Can you work these out from the model? Positions are in its coordinate system, mm. Face numbers are marked on the shaded views. A direction names the side the tool comes from. Give positions to 0.01 mm unless a question says otherwise; leave off trailing zeros. Order: outer loops, then holes, each group sorted by start corner. A loop starts at its lowest first (then second) coordinate and runs counter-clockwise, first axis right, second up. Notation, with made-up numbers: M 39,68 L 61,68 A16 ccw 61,91 Z; hole C 25.25,83 d6. An arc over 180 degrees is marked long. Answer as a JSON object with one key per item and string values.
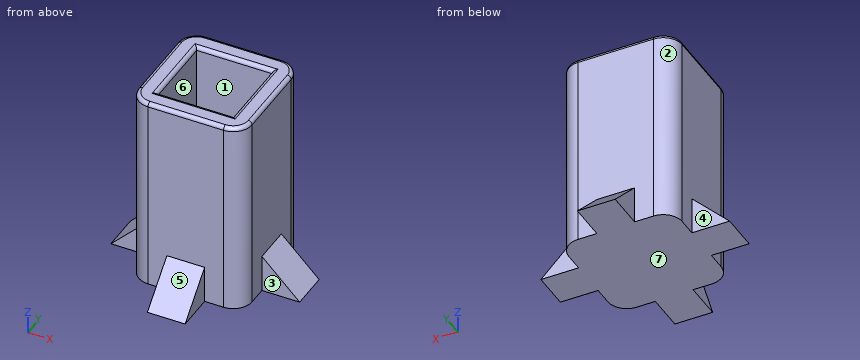
```python
from build123d import *

# Parameters (mm, degrees)
F0_W            = 30
F0_H            = 30
F1_DEPTH        = 3
F2_W            = 30
F2_H            = 30
F2_W_2          = 20
F2_H_2          = 20
F3_DEPTH        = 50
F4_R            = 5
F5_R            = 1
F7_DEPTH        = 5
F7_DEPTH_BACK   = 5
F7_COPIES_COUNT = 4


# Not quite as in the source:
# - a pattern or mirror of a feature is missing from the dataset's text; its kind, count and spacing are read off the source's solid


with BuildPart() as f1:
    # F0 (on Top) → F1 (new body)
    with BuildSketch(Plane.XY):
        Rectangle(F0_W, F0_H)
    extrude(amount=F1_DEPTH)

    # F2 (on face) → F3 (join)
    with BuildSketch(Plane.XY.offset(3)):
        Rectangle(F2_W, F2_H)
        Rectangle(F2_W_2, F2_H_2, mode=Mode.SUBTRACT)
    extrude(amount=F3_DEPTH)

    # F4
    f4_edges = [f1.edges().sort_by_distance(p)[0] for p in [
        (-15, -15, 26.5),
        (-15, 15, 26.5),
        (15, 15, 26.5),
        (15, -15, 26.5),
    ]]
    fillet(f4_edges, radius=F4_R)

    # F5
    f5_edges = [f1.edges().sort_by_distance(p)[0] for p in [
        (15, 0, 53),
        (13.535534, -13.535534, 53),
        (13.535534, 13.535534, 53),
        (0, -15, 53),
        (0, 15, 53),
        (-13.535534, -13.535534, 53),
        (-13.535534, 13.535534, 53),
        (-15, 0, 53),
        (0, 10, 53),
        (10, 0, 53),
        (0, -10, 53),
        (-10, 0, 53),
    ]]
    fillet(f5_edges, radius=F5_R)

    # F6 (on Front) → F7 (join, two sides)
    with BuildSketch(Plane.XZ) as f7_sk:
        Polygon((15, 10), (15, 0), (25, 0), align=None)
    f7 = extrude(amount=F7_DEPTH) + extrude(f7_sk.sketch, amount=-F7_DEPTH_BACK)

    # F7_copies: F7 ×4 about axis
    f7_copies_axis = Axis((0, 0, 0), (0, 0, 1))
    for i in range(1, F7_COPIES_COUNT):
        add(f7.rotate(f7_copies_axis, i * 360 / F7_COPIES_COUNT))


solid = f1.part
```
1) I want a section at C-C on y = 16.5. Write out the boundary of the cut face in (x, z), and give its area (3 significant figures).
Results found:
{"outline": "M -5,0 L 5,0 L 5,8.5 L -5,8.5 Z", "area": "85.0 mm²"}
2) I want a section at A-A on z = 20.5. Write out the boundary of the cut face in (x, y).
Results found:
{"outline": "M -15,-10 A5 ccw -10,-15 L 10,-15 A5 ccw 15,-10 L 15,10 A5 ccw 10,15 L -10,15 A5 ccw -15,10 Z; hole M -10,-10 L 10,-10 L 10,10 L -10,10 Z"}
3) I want a section at D-D on x = 0. Write out the boundary of the cut face in (y, z).
Results found:
{"outline": "M -25,0 L 25,0 L 15,10 L 15,52 A1 ccw 14,53 L 11,53 A1 ccw 10,52 L 10,3 L -10,3 L -10,52 A1 ccw -11,53 L -14,53 A1 ccw -15,52 L -15,10 Z"}
4) Thinking about a two-plate mould opening in Y: for the marked faces 4, 5, 6 and 7, which applies, pulls with the +Y half, pulls with the -Y half, needs draft (parallel to the pull), parting line crosses it, or undercut?
Results found:
{"face 4": "pulls with the +Y half", "face 5": "pulls with the -Y half", "face 6": "undercut", "face 7": "needs draft"}
5) I'm going to push flat-ended pins straight in: pin 1 Ø5 at (x, z) = (-22.5, 5.5) entering from -Y; pin 2 Ø16 at (x, z) = (-1.5, 14) entering from -Y; pin 3 Ø16 at (y, z) = (-0.5, 32.5) entering from +X. Where does each tip first touch, or does it pass through?
Results found:
{"pin 1": "stops at y = -5", "pin 2": "stops at y = -19", "pin 3": "stops at x = 15"}
6) I want a section at B-B on x = -8.5. Write out the boundary of the cut face in (y, z).
Results found:
{"outline": "M -15,0 L 15,0 L 15,52 A1 ccw 14,53 L 11,53 A1 ccw 10,52 L 10,3 L -10,3 L -10,52 A1 ccw -11,53 L -14,53 A1 ccw -15,52 Z"}
7) I need wall thicknesses on L1, parallel to Y at x = -9.5, z = 5; L2, parallel to Z at x = 9, y = -3. Which ranges of each line are inside material? Lowest first, please.
Results found:
{"L1": "y = -15 to -10, 10 to 15", "L2": "z = 0 to 3"}
8) For the marked faces 1, 2 and 3, which set-ups out of +Z, -Z, +X, -X, +Y, -Y let a thin tool reach every point of the face, with its end or its side?
Results found:
{"face 1": "+Z", "face 2": "+Z, -Z, -X, +Y", "face 3": "+Z, -Z, +X, -Y"}
